Input: part model. Units: mm. Frame: model coordinates. A direction names the side the tool comes from. Round coordinates to 2 decimals unless told otherwise and drop trailing zeros. Order: outer loops, then holes, each group sorted by start corner. A loop starts at its lowest first (then second) coordinate and runs counter-clockwise, first axis right, second up. Notation, with made-up numbers: (41.25, 46) -> (58.25, 46) arc R29 ccw to (58.25, 70) -> close; hole circle Ø5 at (21.5, -23.75). An arc over 180 degrees is marked (long way). Answer as CSV lines item,"result". Start each with the question number.
1) Access query for faces 4 (the face through (8.27, -27.12, 2.19)), 5 (the face through (0, 5, 10)). Directions: +Z, -Z, +X, -X, +Y, -Y. A direction counts if a zero-diameter tool reaches every point of the face in a straight line with its end or side. Return the directions, or none.
2) Line query: L1, parallel to Y at x = 17.5, z = 8; L2, parallel to Z at x = 6.5, y = -15; L3, parallel to X at y = -6.5, z = 8. Output: solid intervals per line, ascending.
3) Section query B-B, the plane x = 10. Output: boundary loops of the cut face in (y, z), and give its area (3 significant figures).
4) Section query A-A, the plane z = 10. Output: boundary loops of the cut face in (x, y), and give its area (3 significant figures).
5) Section query C-C, the plane y = -24. Output: boundary loops of the cut face in (x, z).
6) Mould query, pull axis X, two halves, no side actions, for faces 1 (the face through (10.15, 7.32, 9.86)), 2 (the face through (20, 5, 10)), 3 (the face through (10, 4, 20)). Classes: +X half, -X half, draft (parallel to the pull), parting line (faces both ways), or undercut.
7) First-contact query: P1, Ø4, axis at y = -14, z = 16.5, coming from the +X side; P2, Ø10, axis at x = 6.5, y = -7.5, coming from the -Z side; P3, Ø5, axis at x = 18, z = 17, coming from the -Y side; P4, Ø2, axis at x = 4.5, z = 4, coming from the -Y side. Flat tips, straight axial feed; report the tip coordinate or a pass-through.
```python
from build123d import *

# Parameters (mm, degrees)
BOSS_EXTRUDE1_DEPTH = 20
SKETCH2_R           = 8
BOSS_EXTRUDE2_DEPTH = 55


with BuildPart() as part:
    # Sketch1 → Boss-Extrude1 (new body)
    with BuildSketch(Plane.XY):
        with BuildLine():
            Line((0, 10), (0, 0))
            Line((0, 0), (20, 0))
            Line((20, 0), (20, 10))
            ThreePointArc((20, 10), (10, 7.320508076), (0, 10))
        make_face()
    extrude(amount=BOSS_EXTRUDE1_DEPTH)

    # Sketch2 → Boss-Extrude2 (add)
    with BuildSketch(Plane.XZ):
        with Locations((10, 10)):
            Circle(SKETCH2_R)
    extrude(amount=BOSS_EXTRUDE2_DEPTH)


solid = part.part
```
Findings:
1,face 4,"-Y"
1,face 5,"+Z, -Z, -X, +Y, -Y"
2,L1,"y = -55 to 8.78"
2,L2,"z = 2.81 to 17.19"
2,L3,"x = 2.25 to 17.75"
3,outline,"(-55, 2) -> (0, 2) -> (0, 0) -> (7.32, 0) -> (7.32, 20) -> (0, 20) -> (0, 18) -> (-55, 18) -> close"
3,area,"1,030 mm^2"
4,outline,"(0, 0) -> (2, 0) -> (2, -55) -> (18, -55) -> (18, 0) -> (20, 0) -> (20, 10) arc R20 cw to (0, 10) -> close"
4,area,"1,040 mm^2"
5,outline,"circle Ø16 at (10, 10)"
6,face 1,"undercut"
6,face 2,"+X half"
6,face 3,"draft"
7,P1,"stops at x = 16.61"
7,P2,"stops at z = 2"
7,P3,"stops at y = 0"
7,P4,"stops at y = -55"
